from build123d import *

# Parameters (mm, degrees)
SKETCH072_R         = 1.32
PAD047_DEPTH        = 9
POCKET023_DEPTH     = 1.6
HOLE001_D           = 3.3
HOLE001_CSINK_D     = 6
HOLE001_CSINK_ANGLE = 82


with BuildPart() as part:
    # Sketch072 → Pad047 (new body)
    with BuildSketch(Plane.XY):
        Polygon((-7, -51), (5, -51), (5, -21), (-3, -21), (-3, -13.5), (5, -13.5), (5, -5), (-7, -5), align=None)
        with Locations((0, -10)):
            Circle(SKETCH072_R, mode=Mode.SUBTRACT)
    extrude(amount=PAD047_DEPTH)

    # Sketch073 → Pocket023 (cut)
    with BuildSketch(Plane.XY):
        with BuildLine():
            Line((-6, 4), (6, 4))
            Line((6, 4), (6, -21))
            Line((6, -21), (-3, -21))
            Line((-3, -21), (-3, -8))
            ThreePointArc((-3, -8), (-3.87868, -5.87868), (-6, -5))
            Line((-6, -5), (-6, 4))
        make_face()
    extrude(amount=POCKET023_DEPTH, mode=Mode.SUBTRACT)

    # Hole001 (through all)
    with Locations(Plane.XY.offset(9)):
        with Locations((0, -38), (0, -46)):
            CounterSinkHole(HOLE001_D / 2, HOLE001_CSINK_D / 2, counter_sink_angle=HOLE001_CSINK_ANGLE)


solid = part.part
For this review, take the finished solid that the model builds, in its own axes (mm). A direction names the side the tool comes from. Round coordinates to 2 decimals unless told otherwise and drop trailing zeros. Write each loop counter-clockwise with the first axis right and the second up, starting at its lowest first coordinate (ties: lowest second). Pieces come first, ordered by that corner, then holes. Notation, with made-up numbers: (58.5, 68) -> (73.5, 68) arc R3 ccw to (73.5, 73) -> close; hole circle Ø10 at (25.5, 0). An arc over 180 degrees is marked (long way). Use CSV: the item, a comma, the result in double quotes.
(1) To check wall thickness, follow L1, parallel to Y at x = 0, z = 2.5; L2, parallel to X at y = -10, z = 4; L3, parallel to Y at x = -1, z = 3. State the ranges of each line that lie inside material, in increasing order. Write a range as [from, to].
Computed values:
L1,"[-51, -47.65], [-44.35, -39.65], [-36.35, -21], [-13.5, -11.32], [-8.68, -5]"
L2,"[-7, -1.32], [1.32, 5]"
L3,"[-51, -47.31], [-44.69, -39.31], [-36.69, -21], [-13.5, -10.86], [-9.14, -5]"
(2) For faces 4 (the face through (-1, -28, 9)), 5 (the face through (1, -13.5, 5)), 6 (the face through (1, -8, 1.6)), list the 3-axis set-ups (+Z, -Z, +X, -X, +Y, -Y) from which the entire face can be reached by the end or side of a thin tool; tool diameter is ignored.
Computed values:
face 4,"+Z, +X, -X, +Y, -Y"
face 5,"+Z, -Z, +X"
face 6,"-Z, +X, +Y"
(3) Consider section A-A, the plane x = 4. Give the boundary of the cut face in (y, z).
Computed values:
outline,"(-51, 0) -> (-21, 0) -> (-21, 9) -> (-51, 9) -> close; (-13.5, 1.6) -> (-5, 1.6) -> (-5, 9) -> (-13.5, 9) -> close"
(4) Consider section B-B, the plane x = 0. Give the boundary of the cut face in (y, z).
Computed values:
outline,"(-51, 0) -> (-47.65, 0) -> (-47.65, 7.45) -> (-49, 9) -> (-51, 9) -> close; (-44.35, 0) -> (-39.65, 0) -> (-39.65, 7.45) -> (-41, 9) -> (-43, 9) -> (-44.35, 7.45) -> close; (-36.35, 0) -> (-21, 0) -> (-21, 9) -> (-35, 9) -> (-36.35, 7.45) -> close; (-13.5, 1.6) -> (-11.32, 1.6) -> (-11.32, 9) -> (-13.5, 9) -> close; (-8.68, 1.6) -> (-5, 1.6) -> (-5, 9) -> (-8.68, 9) -> close"
(5) Consider section C-C, the plane y = -46. Give the boundary of the cut face in (x, z).
Computed values:
outline,"(-7, 0) -> (-1.65, 0) -> (-1.65, 7.45) -> (-3, 9) -> (-7, 9) -> close; (1.65, 0) -> (5, 0) -> (5, 9) -> (3, 9) -> (1.65, 7.45) -> close"
(6) Draft analysis for pull direction Y (two halves, no side actions). For faces 1 (the face through (-1, -51, 4)), 2 (the face through (5, -36, 4)), 3 (the face through (1, -21, 4)), state which applies: +Y half, -Y half, draft (parallel to the pull), parting line (faces both ways), or undercut.
Computed values:
face 1,"-Y half"
face 2,"draft"
face 3,"undercut"
(7) Clearance check with a flat-ended pin moving along its axis: P1, Ø1, axis at x = 0.5, y = -20, coming from the +Z side. State where the tip first meets the part, or that it passes through.
Computed values:
P1,"through"
(8) Consider section D-D, the plane z = 2.25. Give the boundary of the cut face in (x, y), plus the area to 3 significant figures.
Computed values:
outline,"(-7, -51) -> (5, -51) -> (5, -21) -> (-3, -21) -> (-3, -13.5) -> (5, -13.5) -> (5, -5) -> (-7, -5) -> close; hole circle Ø3.3 at (0, -46); hole circle Ø3.3 at (0, -38); hole circle Ø2.64 at (0, -10)"
area,"469 mm²"
